Input: part model. Units: mm. Frame: model coordinates. Coordinates: 2 decimals unless noted, no trailing zeros. Write each loop counter-clockwise with the first axis right and the second up, starting at its lowest first coordinate (ties: lowest second). Pieces come first, ordered by that corner, then holes. Notation, with made-up numbers: M 11.25,-33 L 67.25,-33 A27 ccw 67.25,-3 Z; hole C 64.5,84 d10. An arc over 180 degrees is marked long. Use one line per item in the form item = value.
from build123d import *

# Parameters (mm, degrees)
SKETCH1_R           = 6.35
BOSS_EXTRUDE1_DEPTH = 177.8
SKETCH2_W           = 38.97891716
SKETCH2_H           = 0.9906
SKETCH3_W           = 26.12692973
SKETCH3_H           = 0.9906
SKETCH4_W           = 46.050080865
SKETCH4_H           = 0.9906
CUT_EXTRUDE1_DEPTH  = 1.778
SKETCH6_W           = 3.175
SKETCH6_H           = 80.766552272
CUT_EXTRUDE2_DEPTH  = 1.778


with BuildPart() as part:
    # Sketch1 → Boss-Extrude1 (new body)
    with BuildSketch(Plane(origin=(0, 0, 0), x_dir=(1, 0, 0), z_dir=(0, 1, 0))):
        Circle(SKETCH1_R)
    extrude(amount=BOSS_EXTRUDE1_DEPTH)

    # Sketch2 → Cut-Revolve1 (revolve, cut)
    with BuildSketch(Plane(origin=(0, 0, 0), x_dir=(0, 0, -1), z_dir=(1, 0, 0))):
        with Locations((-25.43305858, 165.5953)):
            Rectangle(SKETCH2_W, SKETCH2_H)
    revolve(axis=Axis((0, 174.664052397, 0), (0, -1, 0)), mode=Mode.SUBTRACT)

    # Sketch3 → Cut-Revolve2 (revolve, cut)
    with BuildSketch(Plane(origin=(0, 0, 0), x_dir=(0, 0, -1), z_dir=(1, 0, 0))):
        with Locations((-19.007064865, 151.9047)):
            Rectangle(SKETCH3_W, SKETCH3_H)
    revolve(axis=Axis((0, 162.013911259, 0), (0, -1, 0)), mode=Mode.SUBTRACT)

    # Sketch4 → Cut-Revolve3 (revolve, cut)
    with BuildSketch(Plane(origin=(0, 0, 0), x_dir=(0, 0, -1), z_dir=(1, 0, 0))):
        with Locations((-28.968640433, 68.3641)):
            Rectangle(SKETCH4_W, SKETCH4_H)
    revolve(axis=Axis((0, 70.295355643, 0), (0, -1, 0)), mode=Mode.SUBTRACT)

    # Sketch5 → Cut-Extrude1 (cut)
    with BuildSketch(Plane(origin=(6.35, 0, 0), x_dir=(0, 0, -1), z_dir=(1, 0, 0))):
        with BuildLine():
            Line((1.5875, 165.1), (1.5875, 152.4))
            ThreePointArc((1.5875, 152.4), (0, 150.8125), (-1.5875, 152.4))
            Line((-1.5875, 152.4), (-1.5875, 165.1))
            ThreePointArc((-1.5875, 165.1), (0, 166.6875), (1.5875, 165.1))
        make_face()
    extrude(amount=-CUT_EXTRUDE1_DEPTH, mode=Mode.SUBTRACT)

    # Sketch6 → Cut-Extrude2 (cut)
    with BuildSketch(Plane(origin=(6.35, 0, 0), x_dir=(0, 0, -1), z_dir=(1, 0, 0))):
        with Locations((0, 25.301123864)):
            Rectangle(SKETCH6_W, SKETCH6_H)
    extrude(amount=-CUT_EXTRUDE2_DEPTH, mode=Mode.SUBTRACT)


solid = part.part
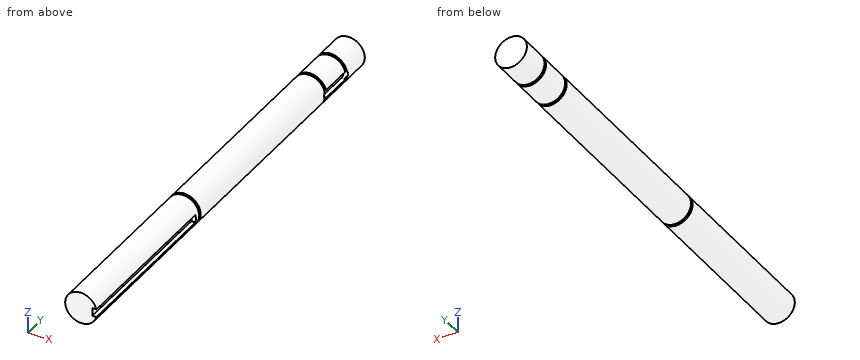
(1) Section query C-C on z = 3.5. Return the cut outline in (x, y).
Computed:
outline = M -5.3,0 L 5.3,0 L 5.3,67.87 L 4.8,67.87 L 4.8,68.86 L 5.3,68.86 L 5.3,151.41 L 4.8,151.41 L 4.8,152.4 L 5.3,152.4 L 5.3,165.1 L 4.8,165.1 L 4.8,166.09 L 5.3,166.09 L 5.3,177.8 L -5.3,177.8 L -5.3,166.09 L -4.8,166.09 L -4.8,165.1 L -5.3,165.1 L -5.3,152.4 L -4.8,152.4 L -4.8,151.41 L -5.3,151.41 L -5.3,68.86 L -4.8,68.86 L -4.8,67.87 L -5.3,67.87 Z
(2) Section query B-B on y = 34. Return the cut outline in (x, z).
Computed:
outline = M 4.57,-1.59 L 4.57,1.59 L 6.15,1.59 A6.35 ccw long 6.15,-1.59 Z
(3) Section query A-A on x = 2.75. Return the cut outline in (y, z), plus the area to 3 significant figures.
Computed:
outline = M 0,-5.72 L 67.87,-5.72 L 67.87,-5.27 L 68.86,-5.27 L 68.86,-5.72 L 151.41,-5.72 L 151.41,-5.27 L 152.4,-5.27 L 152.4,-5.72 L 165.1,-5.72 L 165.1,-5.27 L 166.09,-5.27 L 166.09,-5.72 L 177.8,-5.72 L 177.8,5.72 L 166.09,5.72 L 166.09,5.27 L 165.1,5.27 L 165.1,5.72 L 152.4,5.72 L 152.4,5.27 L 151.41,5.27 L 151.41,5.72 L 68.86,5.72 L 68.86,5.27 L 67.87,5.27 L 67.87,5.72 L 0,5.72 Z
area = 2,030 mm^2
(4) Section query D-D on y = 119.5. Return the cut outline in (x, z), plus the area to 3 significant figures.
Computed:
outline = C 0,0 d12.7
area = 127 mm^2
(5) Line query: probe 1 along Y at (x, z) = (4, 4.5); probe 2 along X at (y, z) = (103, 2.25); probe 3 along X at (y, z) = (111, -0.5). Output: solid intervals per line, ascending.
Computed:
probe_1 = 0 to 67.87, 68.86 to 151.41, 152.4 to 165.1, 166.09 to 177.8
probe_2 = -5.94 to 5.94
probe_3 = -6.33 to 6.33
(6) First-contact query: pin 1 Ø1.3 at (x, y) = (5, 46) entering from -Z; pin 2 Ø4 at (y, z) = (48.5, 0.5) entering from +X; pin 3 Ø2.5 at (y, z) = (156, 0) entering from +X. Flat tips, straight axial feed; report the tip coordinate or a pass-through.
Computed:
pin_1 = -4.63
pin_2 = 6.15
pin_3 = 4.57
